Read the model definition and answer for the solid it produces. Units are mm, in the model's axes. Face numbers are marked on the shaded views. A direction names the side the tool comes from. Give positions to 0.01 mm unless a question says otherwise; leave off trailing zeros. Write each loop counter-clockwise with the first axis right and the second up, starting at its lowest first coordinate (ties: lowest second). Pieces come first, ordered by that corner, then holes. Notation, with made-up numbers: (14, 39.25) -> (71, 39.25) arc R15 cw to (71, 54.25) -> close; hole circle Ø4 at (-22.5, 79). An arc over 180 degrees is marked (long way). Write item = value, one per line.
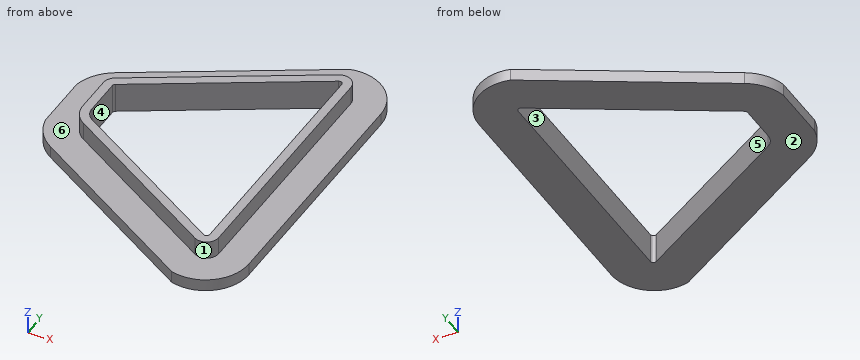
from build123d import *

# Parameters (mm, degrees)
F2_DEPTH = 3
F4_DEPTH = 2
F6_DEPTH = 5.001


with BuildPart() as f2:
    # F1 (on face) → F2 (new body)
    with BuildSketch(Plane.XY):
        with BuildLine():
            ThreePointArc((7.882726, -4.737868), (8.417427, -6.735794), (9.87858, -8.199573))
            Line((9.87858, -8.199573), (37.036658, -23.922675))
            ThreePointArc((37.036658, -23.922675), (39.037693, -23.924472), (40.03873, -22.191823))
            Line((40.03873, -22.191823), (40.03873, -2.183715))
            Line((40.03873, -2.183715), (40.03873, 17.824393))
            ThreePointArc((40.03873, 17.824393), (39.037693, 19.557042), (37.036658, 19.555245))
            Line((37.036658, 19.555245), (8.880653, 3.254395))
            ThreePointArc((8.880653, 3.254395), (8.150077, 2.522506), (7.882726, 1.523543))
            Line((7.882726, 1.523543), (7.882726, -2.183715))
            Line((7.882726, -2.183715), (7.882726, -4.737868))
        make_face()
    extrude(amount=F2_DEPTH)

    # F3 (on face) → F4 (join)
    with BuildSketch(Plane.XY):
        with BuildLine():
            Line((6.51216, -12.028092), (36.024483, -29.11418))
            ThreePointArc((36.024483, -29.11418), (42.238428, -27.868959), (45.03873, -22.183715))
            Line((45.03873, -22.183715), (45.03873, -2.183715))
            Line((45.03873, -2.183715), (45.03873, 17.816285))
            ThreePointArc((45.03873, 17.816285), (42.238428, 23.501529), (36.024483, 24.74675))
            Line((36.024483, 24.74675), (6.51216, 7.660662))
            ThreePointArc((6.51216, 7.660662), (4.133485, 5.486051), (2.882726, 2.515759))
            Line((2.882726, 2.515759), (2.882726, -2.183715))
            Line((2.882726, -2.183715), (2.882726, -6.883189))
            ThreePointArc((2.882726, -6.883189), (4.133485, -9.853481), (6.51216, -12.028092))
        make_face()
    extrude(amount=-F4_DEPTH)

    # F5 (on face) → F6 (cut, through all)
    with BuildSketch(Plane.XY.offset(3)):
        with BuildLine():
            ThreePointArc((9.632207, 1.956256), (9.449563, 1.773284), (9.382726, 1.523543))
            Line((9.382726, 1.523543), (9.382726, -4.737868))
            ThreePointArc((9.382726, -4.737868), (9.716914, -5.986572), (10.630135, -6.901433))
            Line((10.630135, -6.901433), (37.788212, -22.624536))
            ThreePointArc((37.788212, -22.624536), (38.288471, -22.624985), (38.53873, -22.191823))
            Line((38.53873, -22.191823), (38.53873, 17.824393))
            ThreePointArc((38.53873, 17.824393), (38.288471, 18.257555), (37.788212, 18.257106))
            Line((37.788212, 18.257106), (9.632207, 1.956256))
        make_face()
    extrude(amount=-F6_DEPTH, mode=Mode.SUBTRACT)


solid = f2.part
(1) The part is cut by section C-C on y = -11. Determine the outline of the cut face in (x, z).
Checks:
outline = (5.13, -2) -> (17.71, -2) -> (17.71, 3) -> (14.72, 3) -> (14.72, 0) -> (5.13, 0) -> close; (38.54, -2) -> (45.04, -2) -> (45.04, 0) -> (40.04, 0) -> (40.04, 3) -> (38.54, 3) -> close
(2) The part is cut by section D-D on z = 2.35. Determine the outline of the cut face in (x, y), plus the area to 3 significant figures.
Checks:
outline = (7.88, -4.74) arc R4 ccw to (9.88, -8.2) -> (37.04, -23.92) arc R2 ccw to (40.04, -22.19) -> (40.04, 17.82) arc R2 ccw to (37.04, 19.56) -> (8.88, 3.25) arc R2 ccw to (7.88, 1.52) -> close; hole (9.38, -4.74) arc R2.5 ccw to (10.63, -6.9) -> (37.79, -22.62) arc R0.5 ccw to (38.54, -22.19) -> (38.54, 17.82) arc R0.5 ccw to (37.79, 18.26) -> (9.63, 1.96) arc R0.5 ccw to (9.38, 1.52) -> close
area = 180 mm²
(3) Given P1, Ø1, axis at y = 12.5, z = 1, coming from the -X side; P2, Ø2, axis at x = 37.5, y = 9.5, coming from the +Z side; P3, Ø3, axis at x = 33, z = 0, coming from the -Y side; P4, Ø2.5, axis at y = -0.5, z = 2, coming from the -X side, each flat-ended and moving along its own axis, determine where each tip first touches the part or whether it passes through.
Checks:
P1 = 23.99
P2 = through
P3 = -28.23
P4 = 7.88
(4) The part is cut by section B-B on x = 30. Determine the outline of the cut face in (y, z).
Checks:
outline = (-25.63, -2) -> (-18.12, -2) -> (-18.12, 3) -> (-19.85, 3) -> (-19.85, 0) -> (-25.63, 0) -> close; (13.75, -2) -> (21.26, -2) -> (21.26, 0) -> (15.48, 0) -> (15.48, 3) -> (13.75, 3) -> close
(5) The part is cut by section A-A on z = -0.85. Determine the outline of the cut face in (x, y), plus the area to 3 significant figures.
Checks:
outline = (2.88, -6.88) arc R7.53 ccw to (6.51, -12.03) -> (36.02, -29.11) arc R7.17 ccw to (45.04, -22.18) -> (45.04, 17.82) arc R7.17 ccw to (36.02, 24.75) -> (6.51, 7.66) arc R7.53 ccw to (2.88, 2.52) -> close; hole (9.38, -4.74) arc R2.5 ccw to (10.63, -6.9) -> (37.79, -22.62) arc R0.5 ccw to (38.54, -22.19) -> (38.54, 17.82) arc R0.5 ccw to (37.79, 18.26) -> (9.63, 1.96) arc R0.5 ccw to (9.38, 1.52) -> close
area = 887 mm²
(6) Consider L1, parallel to Z at x = 42.5, y = -21.5; L2, parallel to X at y = -5, z = -1.1; L3, parallel to X at y = 11.5, z = 1.5. Determine where each line is inside the solid, lowest interval first.
Checks:
L1 = -2 to 0
L2 = 2.88 to 9.4, 38.54 to 45.04
L3 = 23.12 to 26.12, 38.54 to 40.04
(7) A tool of negligible diameter and unlimited length cuts with its end or side. For the marked faces 5 and 6, from which of +Z, -Z, +X, -X, +Y, -Y can it reach the whole face along a straight path? Write none if from no direction.
Checks:
face_5 = +Z, -Z
face_6 = +Z
(8) For a pull along Y with two mould halves and no side action, classify the marked faces 1, 2, 3 and 4 as released by +Y, released by -Y, zero draft, split by the parting line, or undercut.
Checks:
face_1 = released by -Y
face_2 = zero draft
face_3 = undercut
face_4 = undercut
